Check sheet for the modelled part. Datum: model origin and axes. Units: mm. Face numbers are marked on the shaded views. A direction names the side the tool comes from. Coordinates: 2 decimals unless noted, no trailing zeros. Order: outer loops, then holes, each group sorted by start corner. A loop starts at its lowest first (then second) coordinate and runs counter-clockwise, first axis right, second up.
1. Gauge pin test, flat ends, axial feed: pin 1 Ø1 at (x, y) = (-15, 1.5) entering from +Z; pin 2 Ø3.5 at (x, z) = (19, -0.35) entering from +Y; pin 3 Ø2.5 at (x, y) = (2, 6.5) entering from -Z. Record the tip position at first contact, or that the pin passes through.
2. Cross-section at B-B (x = 12). Enter the section's corners in (y, z), then the cut area to 3 significant figures.
3. Cross-section at C-C (y = 9). Enter the section's corners in (x, z), then the cut area to 3 significant figures.
4. Cross-section at D-D (z = 2). Enter the section's corners in (x, y), then the cut area to 3 significant figures.
5. Set-up check for the marked faces 1 and 2: record each of +Z, -Z, +X, -X, +Y, -Y from which the full face is reachable in a straight line by a thin tool's end or side.
6. Thickness scan on line 1 (Z direction, x = -31, y = 0.95); line 2 (Y direction, x = -2.5, z = -3.25); line 3 (Z direction, x = -19.5, y = 9.75). Record the ranges inside material, lowest first.
7. Cross-section at A-A (x = 19). Enter the section's corners in (y, z), then the cut area to 3 significant figures.
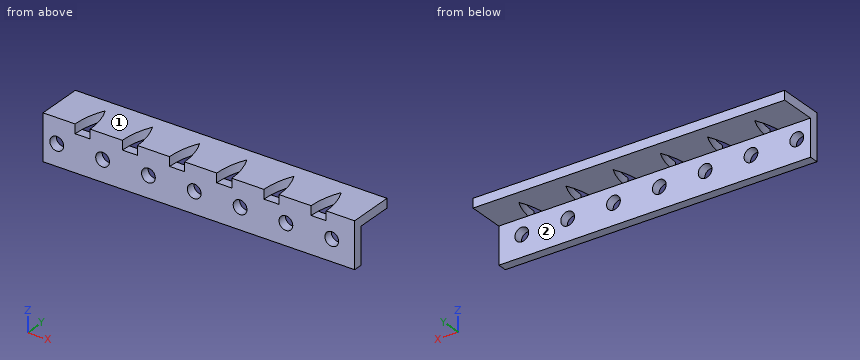
```python
from build123d import *

# Parameters (mm, degrees)
SKETCH1_W                      = 68
SKETCH1_H                      = 10
SKETCH1_R                      = 1.5025
BOSS_EXTRUDE1_DEPTH            = 10
CUT_EXTRUDE1_REACH             = 7
SKETCH2_W                      = 68
SKETCH2_H                      = 8
CUT_EXTRUDE1_DIRECTION_2_DEPTH = 3
CUT_EXTRUDE2_DEPTH             = 2


with BuildPart() as part:
    # Sketch1 → Boss-Extrude1 (new body)
    with BuildSketch(Plane(origin=(0, 0, 0), x_dir=(1, 0, 0), z_dir=(0, 1, 0))):
        Rectangle(SKETCH1_W, SKETCH1_H)
        with Locations((-31, 0.35)):
            Circle(SKETCH1_R, mode=Mode.SUBTRACT)
        with Locations((-21, 0.35)):
            Circle(SKETCH1_R, mode=Mode.SUBTRACT)
        with Locations((-11, 0.35)):
            Circle(SKETCH1_R, mode=Mode.SUBTRACT)
        with Locations((-1, 0.35)):
            Circle(SKETCH1_R, mode=Mode.SUBTRACT)
        with Locations((9, 0.35)):
            Circle(SKETCH1_R, mode=Mode.SUBTRACT)
        with Locations((19, 0.35)):
            Circle(SKETCH1_R, mode=Mode.SUBTRACT)
        with Locations((29, 0.35)):
            Circle(SKETCH1_R, mode=Mode.SUBTRACT)
    extrude(amount=BOSS_EXTRUDE1_DEPTH)

    # Sketch2 → Cut-Extrude1 (cut, up to next)
    with BuildSketch(Plane.XY, mode=Mode.PRIVATE) as cut_extrude1_sk1:
        with Locations((0, 6)):
            Rectangle(SKETCH2_W, SKETCH2_H)
    cut_extrude1_tool1 = extrude(cut_extrude1_sk1.sketch, amount=-CUT_EXTRUDE1_REACH, mode=Mode.PRIVATE) & part.part
    add(cut_extrude1_tool1.solids().sort_by_distance((0, 6, 0))[0], mode=Mode.SUBTRACT)

    # Sketch2 → Cut-Extrude1 direction 2 (cut)
    with BuildSketch(Plane.XY):
        with Locations((0, 6)):
            Rectangle(SKETCH2_W, SKETCH2_H)
    extrude(amount=CUT_EXTRUDE1_DIRECTION_2_DEPTH, mode=Mode.SUBTRACT)

    # Sketch3 → Cut-Extrude2 (cut)
    with BuildSketch(Plane.XY.offset(5)):
        with BuildLine():
            Line((-27, 0), (-23.7, 0))
            add(Edge.make_bspline(
                [(-25.35, 7), (-23.734888234, 3.724961413), (-23.7, 0)],
                knots=[0, 0, 0, 1, 1, 1], degree=2))
            add(Edge.make_bspline(
                [(-25.35, 7), (-26.965111766, 3.724961413), (-27, 0)],
                knots=[0, 0, 0, 1, 1, 1], degree=2))
        make_face()
        with BuildLine():
            Line((-16.7, 0), (-13.4, 0))
            add(Edge.make_bspline(
                [(-15.05, 7), (-13.434888234, 3.724961413), (-13.4, 0)],
                knots=[0, 0, 0, 1, 1, 1], degree=2))
            add(Edge.make_bspline(
                [(-15.05, 7), (-16.665111766, 3.724961413), (-16.7, 0)],
                knots=[0, 0, 0, 1, 1, 1], degree=2))
        make_face()
        with BuildLine():
            Line((-6.4, 0), (-3.1, 0))
            add(Edge.make_bspline(
                [(-4.75, 7), (-3.134888234, 3.724961413), (-3.1, 0)],
                knots=[0, 0, 0, 1, 1, 1], degree=2))
            add(Edge.make_bspline(
                [(-4.75, 7), (-6.365111766, 3.724961413), (-6.4, 0)],
                knots=[0, 0, 0, 1, 1, 1], degree=2))
        make_face()
        with BuildLine():
            Line((3.9, 0), (7.2, 0))
            add(Edge.make_bspline(
                [(5.55, 7), (7.165111766, 3.724961413), (7.2, 0)],
                knots=[0, 0, 0, 1, 1, 1], degree=2))
            add(Edge.make_bspline(
                [(5.55, 7), (3.934888234, 3.724961413), (3.9, 0)],
                knots=[0, 0, 0, 1, 1, 1], degree=2))
        make_face()
        with BuildLine():
            Line((14.2, 0), (17.5, 0))
            add(Edge.make_bspline(
                [(15.85, 7), (17.465111766, 3.724961413), (17.5, 0)],
                knots=[0, 0, 0, 1, 1, 1], degree=2))
            add(Edge.make_bspline(
                [(15.85, 7), (14.234888234, 3.724961413), (14.2, 0)],
                knots=[0, 0, 0, 1, 1, 1], degree=2))
        make_face()
        with BuildLine():
            Line((24.5, 0), (27.8, 0))
            add(Edge.make_bspline(
                [(26.15, 7), (27.765111766, 3.724961413), (27.8, 0)],
                knots=[0, 0, 0, 1, 1, 1], degree=2))
            add(Edge.make_bspline(
                [(26.15, 7), (24.534888234, 3.724961413), (24.5, 0)],
                knots=[0, 0, 0, 1, 1, 1], degree=2))
        make_face()
    extrude(amount=-CUT_EXTRUDE2_DEPTH, mode=Mode.SUBTRACT)


solid = part.part
```
Data:
1. pin 1: stops at z = 3
1. pin 2: stops at y = 2
1. pin 3: stops at z = 3
2. outline: (0, -5) - (2, -5) - (2, 3) - (10, 3) - (10, 5) - (0, 5) - close
2. area: 36.0 mm2
3. outline: (-34, 3) - (34, 3) - (34, 5) - (-34, 5) - close
3. area: 136 mm2
4. outline: (-34, 0) - (34, 0) - (34, 2) - (-34, 2) - close
4. area: 136 mm2
5. face 1: +Z, +X, -X, +Y, -Y
5. face 2: -Z, +X, -X, +Y
6. line 1: z = -5 to -1.85, 1.15 to 5
6. line 2: y = 0 to 2
6. line 3: z = 3 to 5
7. outline: (0, -5) - (2, -5) - (2, -1.85) - (0, -1.85) - close; (0, 1.15) - (2, 1.15) - (2, 3) - (10, 3) - (10, 5) - (0, 5) - close
7. area: 30.0 mm2
